Geometry check sheet. Reference: the model listing, model coordinates, mm. Give positions to 0.01 mm unless a question says otherwise; leave off trailing zeros. Order: outer loops, then holes, each group sorted by start corner. A loop starts at its lowest first (then second) coordinate and runs counter-clockwise, first axis right, second up. Notation, with made-up numbers: (83, 87.5) - (109, 87.5) arc R21 cw to (109, 97.5) - close; hole circle Ø1 at (-1.75, 78). An arc over 180 degrees is marked (long way). Put each result on its own line as item: value. Start each with the question number.
```python
from build123d import *

# Parameters (mm, degrees)
EXTRUSION1_DEPTH = 274.5
ESQUISSE2_R      = 1.5
ESQUISSE2_R_2    = 2
EXTRUSION2_DEPTH = 300
ESQUISSE3_R      = 1.5
EXTRUSION3_DEPTH = 10
ESQUISSE4_W      = 20
ESQUISSE4_H      = 1.5
EXTRUSION4_DEPTH = 5


with BuildPart() as part:
    # Esquisse1 → Extrusion1 (new body)
    with BuildSketch(Plane.XY):
        Polygon((-17.43168638, -13.726631579), (-17.43168638, -15.226631579), (2.56831362, -15.226631579), (2.56831362, 4.773368421), (1.06831362, 4.773368421), (1.06831362, -13.726631579), align=None)
    extrude(amount=EXTRUSION1_DEPTH)

    # Esquisse2 → Extrusion2 (cut)
    with BuildSketch(Plane(origin=(0, -13.726631579, 0), x_dir=(-1, 0, 0), z_dir=(0, 1, 0))):
        with Locations((7.43168638, 204.5)):
            Circle(ESQUISSE2_R)
        with Locations((4.93168638, 4.5)):
            Circle(ESQUISSE2_R_2)
        with Locations((4.93168638, 15.5)):
            Circle(ESQUISSE2_R_2)
        with Locations((4.93168638, 248.5)):
            Circle(ESQUISSE2_R_2)
        with Locations((4.93168638, 259.5)):
            Circle(ESQUISSE2_R_2)
        with Locations((7.43168638, 59.5)):
            Circle(ESQUISSE2_R)
    extrude(amount=-EXTRUSION2_DEPTH, mode=Mode.SUBTRACT)

    # Esquisse3 → Extrusion3 (cut)
    with BuildSketch(Plane(origin=(2.56831362, 0, 0), x_dir=(0, 0, -1), z_dir=(1, 0, 0))):
        with Locations((-266, -5.226631579)):
            Circle(ESQUISSE3_R)
        with Locations((-5, -5.226631579)):
            Circle(ESQUISSE3_R)
        with Locations((-15, -5.226631579)):
            Circle(ESQUISSE3_R)
        with Locations((-59.5, -5.226631579)):
            Circle(ESQUISSE3_R)
        with Locations((-204.5, -5.226631579)):
            Circle(ESQUISSE3_R)
        with Locations((-181.5, -3.726631579)):
            Circle(ESQUISSE3_R)
        with Locations((-138.5, -3.726631579)):
            Circle(ESQUISSE3_R)
    extrude(amount=-EXTRUSION3_DEPTH, mode=Mode.SUBTRACT)

    # Esquisse4 → Extrusion4 (add)
    with BuildSketch(Plane(origin=(0, 0, 0), x_dir=(-1, 0, 0), z_dir=(0, 0, -1))):
        with Locations((7.43168638, -14.476631579)):
            Rectangle(ESQUISSE4_W, ESQUISSE4_H)
    extrude(amount=EXTRUSION4_DEPTH)


solid = part.part
```
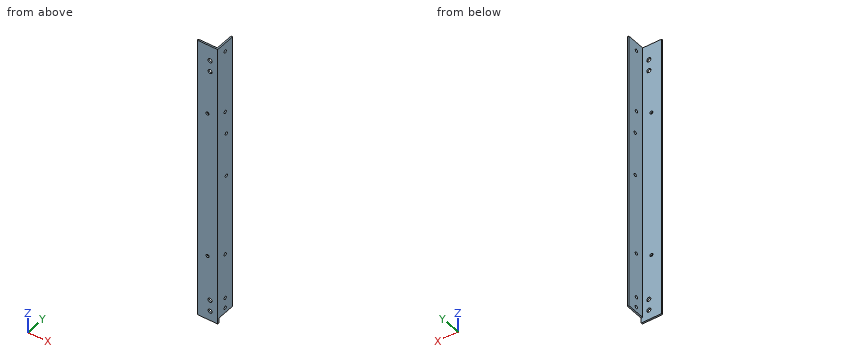
Item 1: Cross-section at C-C (y = -11). Enter the section's corners in (x, z), and give its area (3 significant figures).
Item 2: Gauge pin test, flat ends, axial feed: pin 1 Ø2.5 at (y, z) = (-5.23, 59.5) entering from -X; pin 2 Ø5 at (y, z) = (-5.23, 5) entering from -X; pin 3 Ø5 at (x, z) = (-9, 69) entering from +Y; pin 4 Ø1.2 at (x, y) = (1.5, -3) entering from -Z. Record the tip position at first contact, or that the pin passes through.
Item 3: Cross-section at A-A (x = -11.25). Enter the section's corners in (y, z).
Item 4: Cross-section at B-B (z = 31.5). Enter the section's corners in (x, y), and give its area (4 significant figures).
Item 5: Thickness scan on line 1 along Z through (x, y) = (-4.5, -14.5); line 2 along Y through (x, z) = (-14.5, 82.5); line 3 along X through (y, z) = (1, 108.5). Record the ranges inside material, lowest first.
Recorded:
1. outline: (1.07, 0) - (2.57, 0) - (2.57, 274.5) - (1.07, 274.5) - close
1. area: 412 mm^2
2. pin 1: passes through
2. pin 2: stops at x = 1.07
2. pin 3: stops at y = -13.73
2. pin 4: stops at z = 0
3. outline: (-15.23, -5) - (-13.73, -5) - (-13.73, 274.5) - (-15.23, 274.5) - close
4. outline: (-17.43, -15.23) - (2.57, -15.23) - (2.57, 4.77) - (1.07, 4.77) - (1.07, -13.73) - (-17.43, -13.73) - close
4. area: 57.75 mm^2
5. line 1: z = -5 to 2.55, 6.45 to 13.55, 17.45 to 246.55, 250.45 to 257.55, 261.45 to 274.5
5. line 2: y = -15.23 to -13.73
5. line 3: x = 1.07 to 2.57
